Read the model definition and answer for the solid it produces. Units are mm, in the model's axes. A direction names the side the tool comes from. Coordinates: 2 decimals unless noted, no trailing zeros. Write each loop counter-clockwise with the first axis right and the second up, starting at its lowest first coordinate (ties: lowest second). Pieces come first, ordered by that corner, then holes. Notation, with made-up numbers: M 81,80.25 L 117,80.25 A24 cw 117,112.25 Z; hole C -6,15 d10. An arc over 180 degrees is marked long. Write item = value, one per line.
from build123d import *

# Parameters (mm, degrees)
F0_R        = 12.7
F0_R_2      = 10
F1_DEPTH    = 80
F2_R        = 10
F2_R_2      = 8.75
F3_DEPTH    = 67.056
F3_FACE_R   = 12.7
F3_FACE_R_2 = 8.75
F4_DEPTH    = 19.05


with BuildPart() as f1:
    # F0 (on Top) → F1 (new body)
    with BuildSketch(Plane.XY):
        Circle(F0_R)
        Circle(F0_R_2, mode=Mode.SUBTRACT)
    extrude(amount=F1_DEPTH)

    # F2 (on Top) → F3 (join)
    with BuildSketch(Plane.XY):
        Circle(F2_R)
        Circle(F2_R_2, mode=Mode.SUBTRACT)
    extrude(amount=F3_DEPTH)

    # F3_face (on face) → F4 (join)
    with BuildSketch(Plane(origin=(0, 0, 0), x_dir=(1, 0, 0), z_dir=(0, 0, -1))):
        Circle(F3_FACE_R)
        Circle(F3_FACE_R_2, mode=Mode.SUBTRACT)
    extrude(amount=F4_DEPTH)


solid = f1.part
Item 1: Find section C-C (z = 74). Determine the outline of the cut face in (x, y).
Worked answers:
outline = C 0,0 d25.4; hole C 0,0 d20
Item 2: Consider line 1 along Y through (x, z) = (0.5, 73); line 2 along X through (y, z) = (0, 35). Determine where each line is inside the solid, lowest interval first. Write a range as from..to.
Worked answers:
line_1 = -12.69..-9.99, 9.99..12.69
line_2 = -12.7..-8.75, 8.75..12.7
Item 3: Which of the six approach directions +Z, -Z, +X, -X, +Y, -Y give full straight-line access (tool end or side, diameter ignored) to faces 4 (the face through (-6.944, 5.324, 24.606)), 5 (the face through (-2.17, -9.76, 73.44))?
Worked answers:
face_4 = +Z, -Z
face_5 = +Z
Item 4: For a pull along X with two mould halves and no side action, classify faces 1 (the face through (-2.75, 12.4, 31.17)), 2 (the face through (-0.1, -10.3, 80)), 3 (the face through (0, -9, 67.056)) as released by +X, released by -X, zero draft, split by the parting line, or undercut.
Worked answers:
face_1 = split by the parting line
face_2 = zero draft
face_3 = undercut
Item 5: Flat-ended cylindrical pins translate along their axes: pin 1 (3 mm diameter, centred on y = 3.5, z = 34, fed in from -X); pin 2 (1 mm diameter, centred on x = 1, z = 33.5, fed in from -Y); pin 3 (12 mm diameter, centred on x = 0, y = 0, fed in from -Z). Find the tip coordinate at first contact, or state that the pin passes through.
Worked answers:
pin_1 = -12.54
pin_2 = -12.69
pin_3 = through
Item 6: Find section D-D (z = 33). Determine the outline of the cut face in (x, y).
Worked answers:
outline = C 0,0 d25.4; hole C 0,0 d17.5
Item 7: Find section A-A (y = 0). Determine the outline of the cut face in (x, z).
Worked answers:
outline = M -12.7,-19.05 L -8.75,-19.05 L -8.75,67.06 L -10,67.06 L -10,80 L -12.7,80 Z; M 8.75,-19.05 L 12.7,-19.05 L 12.7,80 L 10,80 L 10,67.06 L 8.75,67.06 Z
